Part model, mm, in its own coordinate system. Face numbers are marked on the shaded views. A direction names the side the tool comes from. Give positions to 0.01 mm unless a question says otherwise; leave off trailing zeros. Order: outer loops, then holes, each group sorted by start corner. A loop starts at its lowest first (then second) coordinate and runs counter-clockwise, first axis right, second up. Notation, with made-up numbers: M 34,49 L 87,49 A18 ccw 87,82 Z; hole C 23.25,67 d9. An arc over 180 degrees is marked long. Return JSON: item names as keys, results as strings.
from build123d import *

# Parameters (mm, degrees)
F0_R     = 10
F1_DEPTH = 42
F2_R     = 16.4716554
F2_R_2   = 4
F3_DEPTH = 6
F5_D     = 6.8
F5_DEPTH = 25
F5_TIP   = 2.0429261047


with BuildPart() as f1:
    # F0 (on Front) → F1 (new body)
    with BuildSketch(Plane.XZ):
        Circle(F0_R)
    extrude(amount=-F1_DEPTH)

    # F2 (on face) → F3 (cut)
    with BuildSketch(Plane.XZ):
        Circle(F2_R)
        Circle(F2_R_2, mode=Mode.SUBTRACT)
    extrude(amount=-F3_DEPTH, mode=Mode.SUBTRACT)

    # F5
    with Locations(Plane(origin=(0, 42, 0), x_dir=(-1, 0, 0), z_dir=(0, 1, 0))):
        with Locations((0, 0)):
            Hole(F5_D / 2, depth=F5_DEPTH)
            with Locations((0, 0, -(F5_DEPTH + F5_TIP / 2))):  # 118° drill point
                Cone(0, F5_D / 2, F5_TIP, mode=Mode.SUBTRACT)


solid = f1.part
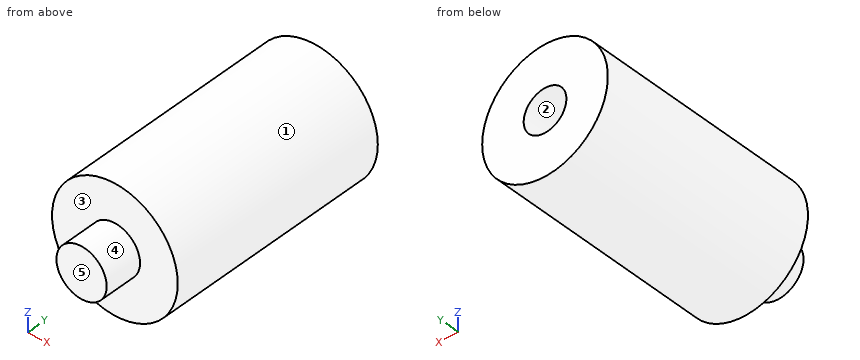
Q1. Band-saw the part on C-C (x = 5.25). Give the cut face in (y, z), then the cut area to 3 significant figures.
Established:
{"outline": "M 6,-8.51 L 42,-8.51 L 42,8.51 L 6,8.51 Z", "area": "613 mm²"}
Q2. Two-plate mould, pull along X, no slides. Class the marked faces 1, 2 and 3: +X half, -X half, draft (parallel to the pull), parting line (faces both ways), or undercut.
Established:
{"face 1": "parting line", "face 2": "undercut", "face 3": "draft"}
Q3. Band-saw the part on A-A (y = 27). Give the cut face in (x, z).
Established:
{"outline": "C 0,0 d20; hole C 0,0 d6.8"}
Q4. Band-saw the part on B-B (z = 6). Give the cut face in (x, y).
Established:
{"outline": "M -8,6 L 8,6 L 8,42 L -8,42 Z"}
Q5. Probe line 1 along X through (y, z) = (34.5, -0.25); line 2 along Z through (x, y) = (0, 23); line 3 along Y through (x, z) = (-9, 2). List the from-to ranges inside material, lowest first.
Established:
{"line 1": "x = -10 to -3.39, 3.39 to 10", "line 2": "z = -10 to -3.4, 3.4 to 10", "line 3": "y = 6 to 42"}
Q6. 3-axis set-ups, long thin cutter, end or side, ignore diameter. For the marked faces 4 and 5: which of +Z, -Z, +X, -X, +Y, -Y reach the whole face in a straight line?
Established:
{"face 4": "-Y", "face 5": "+Z, -Z, +X, -X, -Y"}
Q7. Pin check, flat tips, straight feed: pin 1 (1 mm diameter, centred on y = 21.5, z = -6.5, fed in from +X); pin 2 (3 mm diameter, centred on x = -5.5, z = -3.5, fed in from -Y); pin 3 (3 mm diameter, centred on x = -4.5, y = 19, fed in from +Z). Stop position of each tip, or through.
Established:
{"pin 1": "stops at x = 8", "pin 2": "stops at y = 6", "pin 3": "stops at z = 9.54"}
